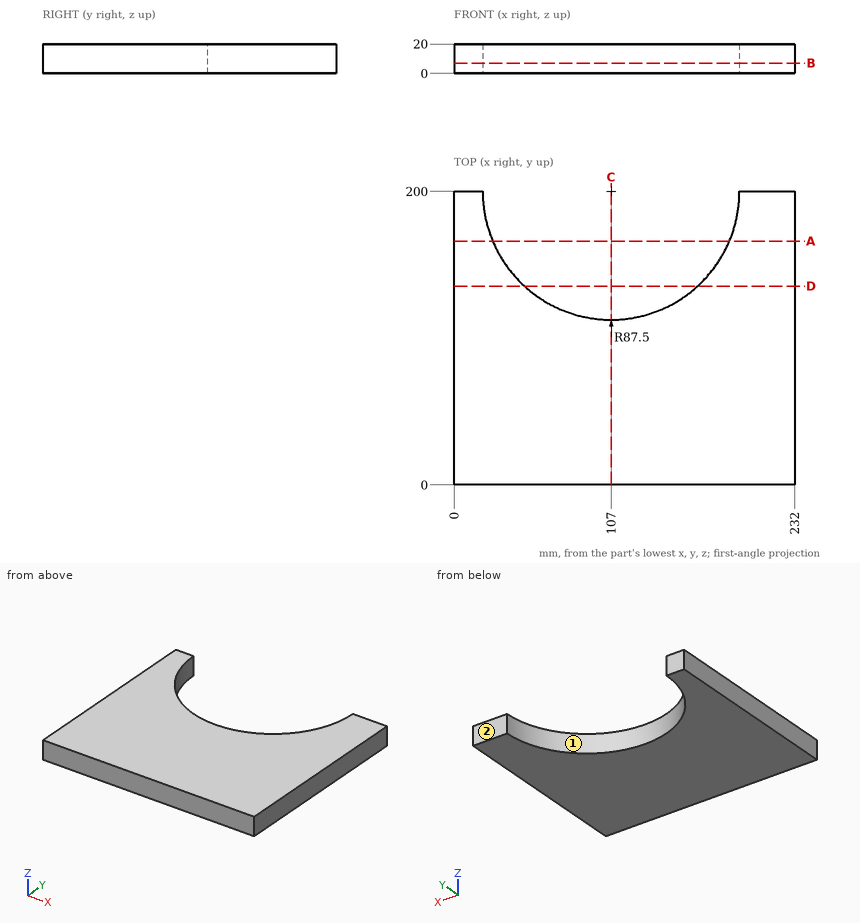
Input: dimensioned drawing with shaded views. Units: mm. Origin: part minimum x, y, z. Round coordinates to 2 decimals unless told otherwise and drop trailing zeros. Loops run counter-clockwise (first coordinate to the right, second up) from the corner with the lowest first, then second, coordinate; pieces in that order, holes last. Notation, with made-up numbers: (-24, 42) -> (33, 42) arc R27 cw to (33, 73) -> close; hole circle Ø9 at (8, -2.75). An arc over 180 degrees is marked (long way). One line per item, written item: value.
(1) Mould query, pull axis X, two halves, no side actions, for the marked faces 1 and 2. Classes: pulls with the +X half, pulls with the -X half, needs draft (parallel to the pull), parting line crosses it, or undercut.
Geometry check:
face 1: undercut
face 2: needs draft
(2) Material intervals for line 1 (X direction, y = 174, z = 11.25); line 2 (X direction, y = 178, z = 13.25); line 3 (Y direction, x = 113, z = 3.5), sorted ascending. Write a range as [from, to].
Geometry check:
line 1: [0, 23.45], [190.55, 232]
line 2: [0, 22.31], [191.69, 232]
line 3: [0, 112.71]
(3) Section A-A (y = 166). Return the cut outline in (x, z).
Geometry check:
outline: (0, 0) -> (26.38, 0) -> (26.38, 20) -> (0, 20) -> close; (187.62, 0) -> (232, 0) -> (232, 20) -> (187.62, 20) -> close
(4) Pin query (flat end, axial travel): pin 1 (4 mm diameter, centred on y = 25.5, z = 2.5, fed in from -X). Return the tip coordinate at first contact, or that it passes through.
Geometry check:
pin 1: x = 0
(5) Section D-D (y = 135.5). Return the cut outline in (x, z).
Geometry check:
outline: (0, 0) -> (47.87, 0) -> (47.87, 20) -> (0, 20) -> close; (166.13, 0) -> (232, 0) -> (232, 20) -> (166.13, 20) -> close
(6) Section C-C (x = 107). Return the cut outline in (y, z).
Geometry check:
outline: (0, 0) -> (112.5, 0) -> (112.5, 20) -> (0, 20) -> close
(7) Section B-B (z = 7). Return the cut outline in (x, y), plus the area to 3 significant figures.
Geometry check:
outline: (0, 0) -> (232, 0) -> (232, 200) -> (194.5, 200) arc R87.5 cw to (19.5, 200) -> (0, 200) -> close
area: 34,400 mm2
